Build history of the part. All positions in model axes, mm. Give positions to 0.01 mm unless a question says otherwise; leave off trailing zeros. Order: outer loops, then holes, each group sorted by start corner. A loop starts at its lowest first (then second) coordinate and runs counter-clockwise, first axis right, second up. Notation, with made-up numbers: (55.5, 23) - (67.5, 23) arc R34 cw to (67.5, 59) - close; hole circle Ø3 at (-16, -40). An arc over 180 degrees is marked (long way). Answer in a Markdown table with one row per item.
Autodesk Fusion 360 part; units mm, degrees
sketch "Sketch1" plane through (0, 0, 0) normal (0, 0, 1) x (1, 0, 0)
  circle A0 centre (0, 0) radius 2.8
  circle A1 centre (0, 0) radius 5.5
  dimension "d1" = 5.6
  dimension "d2" = 2.7
extrude "Extrude1" add sketch "Sketch1" along normal blind 4
chamfer "Chamfer1" distance 0.6 angle 45 1 edges at (-2.6105, 1.0125, 0)
fillet "Fillet1" radius 0.8 1 faces at (4.5691, -0.4124, 4)
1. Two-plate mould, pull along Y, no slides. Class faces 1 (the face through (-2.8, -0.1, 1.9)), 2 (the face through (-1.19, 5.37, 1.58)), 3 (the face through (2, 3, 0)): +Y half, -Y half, draft (parallel to the pull), parting line (faces both ways), or undercut.
Check result:
| item | result |
|---|---|
| face 1 | undercut |
| face 2 | parting line |
| face 3 | draft |
2. Probe line 1 (Y direction, x = 0, z = 2.15); line 2 (X direction, y = 2.5, z = 0.85); line 3 (X direction, y = 1.5, z = 1.35). List the from-to ranges inside material, lowest first.
Check result:
| item | result |
|---|---|
| line 1 | y = -5.5 to -2.8, 2.8 to 5.5 |
| line 2 | x = -4.9 to -1.26, 1.26 to 4.9 |
| line 3 | x = -5.29 to -2.36, 2.36 to 5.29 |
3. Cut at A-A on y = 0. Write the cut outline in (x, z).
Check result:
| item | result |
|---|---|
| outline | (-5.5, 0) - (-3.4, 0) - (-2.8, 0.6) - (-2.8, 3.2) arc R0.8 ccw to (-3.6, 4) - (-4.7, 4) arc R0.8 ccw to (-5.5, 3.2) - close; (2.8, 0.6) - (3.4, 0) - (5.5, 0) - (5.5, 3.2) arc R0.8 ccw to (4.7, 4) - (3.6, 4) arc R0.8 ccw to (2.8, 3.2) - close |
4. Cut at C-C on z = 1.5. Write the cut outline in (x, y), and give its area (3 significant figures).
Check result:
| item | result |
|---|---|
| outline | circle Ø11 at (0, 0); hole circle Ø5.6 at (0, 0) |
| area | 70.4 mm² |
